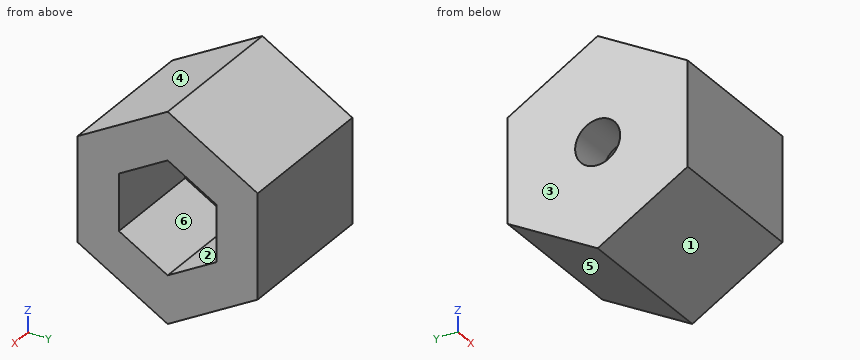
from build123d import *

# Parameters (mm, degrees)
EXTRUDE_1_DEPTH     = 10
CUT_EXTRUDE_1_DEPTH = 7
SKETCH_3_R          = 1.5
CUT_EXTRUDE_2_DEPTH = 7


with BuildPart() as part:
    # 草图1 → 凸台-拉伸1 (new body)
    with BuildSketch(Plane(origin=(0, 0, 0), x_dir=(0, 0, -1), z_dir=(1, 0, 0))):
        Polygon((6.92820323, 0), (3.464101615, 6), (-3.464101615, 6), (-6.92820323, 0), (-3.464101615, -6), (3.464101615, -6), align=None)
    extrude(amount=EXTRUDE_1_DEPTH)

    # 草图2 → 切除-拉伸1 (cut)
    with BuildSketch(Plane(origin=(10, 0, 0), x_dir=(0, 0, -1), z_dir=(1, 0, 0))):
        Polygon((3.75277675, 0), (1.876388375, 3.25), (-1.876388375, 3.25), (-3.75277675, 0), (-1.876388375, -3.25), (1.876388375, -3.25), align=None)
    extrude(amount=-CUT_EXTRUDE_1_DEPTH, mode=Mode.SUBTRACT)

    # 草图3 → 切除-拉伸2 (cut)
    with BuildSketch(Plane(origin=(3, 0, 0), x_dir=(0, 0, -1), z_dir=(1, 0, 0))):
        Circle(SKETCH_3_R)
    extrude(amount=-CUT_EXTRUDE_2_DEPTH, mode=Mode.SUBTRACT)


solid = part.part
Can you work these out from the model? Positions are in its coordinate system, mm. Face numbers are marked on the shaded views. A direction names the side the tool comes from. Round coordinates to 2 decimals unless told otherwise and drop trailing zeros. Order: outer loops, then holes, each group sorted by start corner. A loop starts at its lowest first (then second) coordinate and runs counter-clockwise, first axis right, second up. Notation, with made-up numbers: (77, -17.75) -> (104, -17.75) arc R12 cw to (104, -7.75) -> close; hole circle Ø8 at (-22.5, 40.5). An arc over 180 degrees is marked (long way). Write each question's results on one line, items separated by ' | '. Start each with the question number.
Item 1: If we section it at D-D, the plane z = -3: Write out the boundary of the cut face in (x, y).
Item 2: If we section it at A-A, the plane z = 0: Write out the boundary of the cut face in (x, y).
Item 3: If we section it at B-B, the plane x = 6.75: Write out the boundary of the cut face in (y, z).
Item 4: Which directions (+Z, -Z, +X, -X, +Y, -Y) give clear straight access to the entire face, cutting with the end or side of a thin tool? Please do the marked faces 5 and 6.
Item 5: If we section it at C-C, the plane y = -1.25: Write out the boundary of the cut face in (x, z).
Item 6: Please list where these lines run through material, in increasing order: L1, parallel to Y at x = 1.4, z = 0; L2, parallel to Y at x = 5.75, z = -1; L3, parallel to X at y = 2.25, z = 1.
Item 7: Thinking about a two-plate mould opening in Z: for the marked faces 1, 2, 3 and 4, which applies, +Z half, -Z half, draft (parallel to the pull), parting line (faces both ways), or undercut?
Item 8: Will these pins go through, and if not, where does the flat tip stop? pin 1 (1.5 mm diameter, centred on x = 2.5, y = 1.5, fed in from -Z); pin 2 (2 mm diameter, centred on y = 0.5, z = 0.5, fed in from +X).
Results:
1) outline: (0, -6) -> (10, -6) -> (10, -1.3) -> (3, -1.3) -> (3, 1.3) -> (10, 1.3) -> (10, 6) -> (0, 6) -> close
2) outline: (0, -6) -> (10, -6) -> (10, -3.25) -> (3, -3.25) -> (3, -1.5) -> (0, -1.5) -> close; (0, 1.5) -> (3, 1.5) -> (3, 3.25) -> (10, 3.25) -> (10, 6) -> (0, 6) -> close
3) outline: (-6, -3.46) -> (0, -6.93) -> (6, -3.46) -> (6, 3.46) -> (0, 6.93) -> (-6, 3.46) -> close; hole (-3.25, -1.88) -> (0, -3.75) -> (3.25, -1.88) -> (3.25, 1.88) -> (0, 3.75) -> (-3.25, 1.88) -> close
4) face 5: -Z, +X, -X, +Y | face 6: +X
5) outline: (0, -6.21) -> (10, -6.21) -> (10, -3.03) -> (3, -3.03) -> (3, -0.83) -> (0, -0.83) -> close; (0, 0.83) -> (3, 0.83) -> (3, 3.03) -> (10, 3.03) -> (10, 6.21) -> (0, 6.21) -> close
6) L1: y = -6 to -1.5, 1.5 to 6 | L2: y = -6 to -3.25, 3.25 to 6 | L3: x = 0 to 3
7) face 1: -Z half | face 2: undercut | face 3: draft | face 4: +Z half
8) pin 1: stops at z = -6.5 | pin 2: stops at x = 3
